from build123d import *

# Parameters (mm, degrees)
BASE_EXTRUDE_DEPTH = 12.7
CIRPATTERN1_COUNT  = 2
CIRPATTERN1_ANGLE  = 90


with BuildPart() as part:
    # Sketch1 → Base-Extrude (new, symmetric)
    with BuildSketch(Plane(origin=(-20.32, 17.78, 0), x_dir=(1, 0, 0), z_dir=(0, 0, 1))):
        with BuildLine():
            Line((17.3228, 17.075886512), (19.412382578, 19.800133504))
            ThreePointArc((19.412382578, 19.800133504), (18.838545845, 21.346344632), (17.3228, 21.9964))
            Line((17.3228, 21.9964), (14.38577367, 21.9964))
            ThreePointArc((14.38577367, 21.9964), (12.906383481, 21.383616519), (12.2936, 19.90422633))
            Line((12.2936, 19.90422633), (12.2936, 15.61465))
            Line((12.2936, 15.61465), (10.795, 15.61465))
            Line((10.795, 15.61465), (10.795, 19.90422633))
            ThreePointArc((10.795, 19.90422633), (11.846713258, 22.443286742), (14.38577367, 23.495))
            Line((14.38577367, 23.495), (17.3228, 23.495))
            ThreePointArc((17.3228, 23.495), (20.097934554, 22.182884653), (20.844928673, 19.2054666))
            Line((20.844928673, 19.2054666), (18.8214, 16.567335923))
            Line((18.8214, 16.567335923), (18.8214, 11.485729415))
            Line((18.8214, 11.485729415), (20.32, 9.8028125))
            Line((20.32, 9.8028125), (20.32, -5.180962694))
            Line((20.32, -5.180962694), (19.1389, -6.507329415))
            Line((19.1389, -6.507329415), (19.1389, -12.757931546))
            Line((19.1389, -12.757931546), (20.424084837, -14.043116383))
            ThreePointArc((20.424084837, -14.043116383), (18.821804006, -17.54486751), (15.019825564, -16.932883251))
            ThreePointArc((15.019825564, -16.932883251), (13.348875824, -16.363652979), (12.29528328, -17.78))
            Line((12.29528328, -17.78), (-12.61278328, -17.78))
            ThreePointArc((-12.61278328, -17.78), (-13.666375824, -16.363652979), (-15.337325564, -16.932883251))
            ThreePointArc((-15.337325564, -16.932883251), (-19.047442105, -18.270236732), (-20.870958003, -14.773342558))
            Line((-20.870958003, -14.773342558), (-19.4564, -13.358784555))
            Line((-19.4564, -13.358784555), (-19.4564, -6.507329415))
            Line((-19.4564, -6.507329415), (-20.955, -4.8244125))
            Line((-20.955, -4.8244125), (-20.955, 9.0662125))
            Line((-20.955, 9.0662125), (-19.4564, 10.749129415))
            Line((-19.4564, 10.749129415), (-19.4564, 15.830735923))
            Line((-19.4564, 15.830735923), (-21.479928673, 18.4688666))
            ThreePointArc((-21.479928673, 18.4688666), (-20.732934554, 21.446284653), (-17.9578, 22.7584))
            Line((-17.9578, 22.7584), (-15.02077367, 22.7584))
            ThreePointArc((-15.02077367, 22.7584), (-12.481713258, 21.706686742), (-11.43, 19.16762633))
            Line((-11.43, 19.16762633), (-11.43, 15.61465))
            Line((-11.43, 15.61465), (-12.9286, 15.61465))
            Line((-12.9286, 15.61465), (-12.9286, 19.16762633))
            ThreePointArc((-12.9286, 19.16762633), (-13.541383481, 20.647016519), (-15.02077367, 21.2598))
            Line((-15.02077367, 21.2598), (-17.9578, 21.2598))
            ThreePointArc((-17.9578, 21.2598), (-19.473545845, 20.609744632), (-20.047382578, 19.063533504))
            Line((-20.047382578, 19.063533504), (-17.9578, 16.339286512))
            Line((-17.9578, 16.339286512), (-17.9578, 10.17860201))
            Line((-17.9578, 10.17860201), (-19.4564, 8.495685095))
            Line((-19.4564, 8.495685095), (-19.4564, -4.253885095))
            Line((-19.4564, -4.253885095), (-17.9578, -5.93680201))
            Line((-17.9578, -5.93680201), (-17.9578, -13.979525))
            Line((-17.9578, -13.979525), (-19.4564, -15.478125))
            ThreePointArc((-19.4564, -15.478125), (-18.409738669, -16.906954381), (-16.731785827, -16.33992034))
            ThreePointArc((-16.731785827, -16.33992034), (-14.14499029, -14.797667818), (-11.524190259, -16.2814))
            Line((-11.524190259, -16.2814), (11.206690259, -16.2814))
            ThreePointArc((11.206690259, -16.2814), (13.441553644, -14.818250812), (15.956217628, -15.719297395))
            ThreePointArc((15.956217628, -15.719297395), (17.836242029, -16.3415136), (19.00315301, -14.741525))
            Line((19.00315301, -14.741525), (17.6403, -13.37867199))
            Line((17.6403, -13.37867199), (17.6403, -5.93680201))
            Line((17.6403, -5.93680201), (18.8214, -4.610435289))
            Line((18.8214, -4.610435289), (18.8214, 9.232285095))
            Line((18.8214, 9.232285095), (17.3228, 10.91520201))
            Line((17.3228, 10.91520201), (17.3228, 17.075886512))
        make_face()
    base_extrude = extrude(amount=BASE_EXTRUDE_DEPTH, both=True)

    # CirPattern1: Base-Extrude ×2 about axis
    cirpattern1_axis = Axis((0, 0, 0), (0, 0, 1))
    for i in range(1, CIRPATTERN1_COUNT):
        add(base_extrude.rotate(cirpattern1_axis, i * CIRPATTERN1_ANGLE / (CIRPATTERN1_COUNT - 1)))


solid = part.part
Source: CAD feature listing. Evaluate the final solid. Frame: model axes, mm. A direction names the side the tool comes from. Round coordinates to 2 decimals unless told otherwise and drop trailing zeros. Write each loop counter-clockwise with the first axis right and the second up, starting at its lowest first coordinate (ties: lowest second). Pieces come first, ordered by that corner, then holes. Notation, with made-up numbers: (1, 50.5) - (24, 50.5) arc R7 cw to (24, 54.5) - close; hole circle Ø8 at (35, 71.5). An arc over 180 degrees is marked (long way). Use CSV: the item, a comma, the result in double quotes. Start each with the question number.
(1) First-contact query: pin 1 Ø1.9 at (y, z) = (9, 1) entering from +X; pin 2 Ø1.6 at (x, z) = (-8.5, -3) entering from -Y; pin 3 Ø2 at (y, z) = (36, 1) entering from -X; pin 4 Ø3.5 at (x, z) = (-10.5, -0.5) entering from -Y. Flat tips, straight axial feed; report the tip coordinate or a pass-through.
(2) Material intervals for probe 1 along Y at (x, z) = (-22.5, -2.5) (3 decimals); probe 2 along X at (y, z) = (35, -0.25) (3 decimals); probe 3 along Y at (x, z) = (-8.5, 4), sorted ascending. Write a range as [from, to].
(3) Mould query, pull axis X, two halves, no side actions, for faces 1 (the face through (-1.408, -33.961, 0.178)), 2 (the face through (-33.395, -9, 0)), 3 (the face through (-40.538, -37, 0)). Classes: pulls with the +X half, pulls with the -X half, needs draft (parallel to the pull), parting line crosses it, or undercut.
(4) Cut plane C-C, the plane z = -4.5. Give the number of separate pieces and of enclosed holes in the cut face, and give its area (3 significant figures).
(5) Cut plane B-B, the plane x = -19. Return loops of the section in (y, z) (3 decimals).
(6) Cut plane A-A, the plane y = 21.5. Return loops of the section in (x, z) (3 decimals).
(7) Set-up query: faces 4 (the face through (-41.275, 20, 0)), 5 (the face through (-36, -9.525, 0)), 6 (the face through (-4, 39.776, 0)), 7 (the face through (-31.75, 35, 0)), 8 (the face through (-8, -39.776, 0)). Return all of +Z, -Z, +X, -X, +Y, -Y with unobstructed straight access to the full face (end or side cutting, diameter ignored); none if empty.
Geometry says:
1,pin 1,"x = -1.18"
1,pin 2,"y = -39.78"
1,pin 3,"x = -41.87"
1,pin 4,"y = -40.65"
2,probe 1,"[-41.275, -39.776], [-1.499, 1.499]"
2,probe 2,"[-40.842, -38.953], [-33.249, -31.75], [-9.525, -8.026], [-2.887, -0.998]"
2,probe 3,"[-39.78, -38.28], [-2.68, -1.18], [0, 2.24], [33.39, 40.2]"
3,face 1,"pulls with the +X half"
3,face 2,"undercut"
3,face 3,"pulls with the -X half"
4,separate pieces,"1"
4,enclosed holes,"2"
4,area,"448 mm²"
5,outline,"(-41.275, -12.7) - (-39.776, -12.7) - (-39.776, 12.7) - (-41.275, 12.7) - close; (-1.499, -12.7) - (1.499, -12.7) - (1.499, 12.7) - (-1.499, 12.7) - close"
6,outline,"(-41.275, -12.7) - (-39.776, -12.7) - (-39.776, 12.7) - (-41.275, 12.7) - close; (-1.499, -12.7) - (0, -12.7) - (0, 12.7) - (-1.499, 12.7) - close"
7,face 4,"+Z, -Z, -X, -Y"
7,face 5,"+Z, -Z, -X"
7,face 6,"+Z, -Z"
7,face 7,"+Z, -Z, +Y"
7,face 8,"+Z, -Z, -Y"
